Build history of the part. All positions in model axes, mm. Face numbers are marked on the shaded views. A direction names the side the tool comes from. Give positions to 0.01 mm unless a question says otherwise; leave off trailing zeros. Loops run counter-clockwise (first coordinate to the right, second up) from the corner with the lowest first, then second, coordinate; pieces in that order, holes last. Notation, with made-up numbers: (-33.5, 4.5) -> (14.5, 4.5) arc R26 ccw to (14.5, 24.5) -> close; hole circle Ø4 at (77, -1). An arc over 180 degrees is marked (long way). Answer in a Markdown table with one row per item. Add a question column.
from build123d import *

# Parameters (mm, degrees)
DODANIE_WYCI_GNI_CIE4_DEPTH = 13
SZKIC4_W                    = 21
SZKIC4_H                    = 13
DODANIE_WYCI_GNI_CIE5_DEPTH = 2
SZKIC5_W                    = 21
SZKIC5_H                    = 13
SZKIC5_R                    = 3
DODANIE_WYCI_GNI_CIE6_DEPTH = 4
DODANIE_WYCI_GNI_CIE7_START = -4
SZKIC5_4_R                  = 3
DODANIE_WYCI_GNI_CIE7_DEPTH = 3.6
ZAOKR_GLENIE3_R             = 8


with BuildPart() as part:
    # Szkic3 → Dodanie-wyci_gni_cie4 (new body)
    with BuildSketch(Plane(origin=(0, 0, 0), x_dir=(1, 0, 0), z_dir=(0, 1, 0))):
        Polygon((7.923824764, -2), (7.923824764, -0.6), (5.016097838, -0.6), (2.807764504, 1.65), (-3.360114975, 1.65), (-5.568448309, -0.6), (-8.476175236, -0.6), (-8.476175236, -2), (-10.5, -2), (-10.5, 2), (10.5, 2), (10.5, -2), align=None)
    extrude(amount=DODANIE_WYCI_GNI_CIE4_DEPTH)

    # Szkic4 → Dodanie-wyci_gni_cie5 (add)
    with BuildSketch(Plane(origin=(0, 0, -2), x_dir=(-1, 0, 0), z_dir=(0, 0, -1))):
        with Locations((0, 6.5)):
            Rectangle(SZKIC4_W, SZKIC4_H)
    extrude(amount=DODANIE_WYCI_GNI_CIE5_DEPTH)

    # Szkic5 → Dodanie-wyci_gni_cie6 (add)
    with BuildSketch(Plane(origin=(0, 0, -4), x_dir=(-1, 0, 0), z_dir=(0, 0, -1))):
        with Locations((0, 19.5)):
            Rectangle(SZKIC5_W, SZKIC5_H)
        with Locations((0, 20)):
            Circle(SZKIC5_R, mode=Mode.SUBTRACT)
        with Locations((0, -6.5)):
            Rectangle(SZKIC5_W, SZKIC5_H)
        with Locations((0, -7)):
            Circle(SZKIC5_R, mode=Mode.SUBTRACT)
    extrude(amount=-DODANIE_WYCI_GNI_CIE6_DEPTH)

    # Szkic5_4 → Dodanie-wyci_gni_cie7 (add)
    with BuildSketch(Plane(origin=(0, 0, -4), x_dir=(-1, 0, 0), z_dir=(0, 0, -1)).offset(DODANIE_WYCI_GNI_CIE7_START)):
        with BuildLine():
            Line((3, 16), (-3, 16))
            ThreePointArc((-3, 16), (0, 15), (3, 16))
        make_face()
        with BuildLine():
            ThreePointArc((5, 20), (-2.236067977, 24.472135955), (-3, 16))
            Line((-3, 16), (3, 16))
            ThreePointArc((3, 16), (4.472135955, 17.763932023), (5, 20))
        make_face()
        with Locations((0, 20)):
            Circle(SZKIC5_4_R, mode=Mode.SUBTRACT)
        with BuildLine():
            Line((-3, -3), (3, -3))
            ThreePointArc((3, -3), (0, -2), (-3, -3))
        make_face()
        with BuildLine():
            ThreePointArc((5, -7), (4.472135955, -4.763932023), (3, -3))
            Line((3, -3), (-3, -3))
            ThreePointArc((-3, -3), (-2.236067977, -11.472135955), (5, -7))
        make_face()
        with Locations((0, -7)):
            Circle(SZKIC5_4_R, mode=Mode.SUBTRACT)
    extrude(amount=-DODANIE_WYCI_GNI_CIE7_DEPTH)

    # Zaokr_glenie3
    zaokr_glenie3_edges = [part.edges().sort_by_distance(p)[0] for p in [
        (-10.5, -13, -2),
        (10.5, -13, -2),
        (10.5, 26, -2),
        (-10.5, 26, -2),
    ]]
    fillet(zaokr_glenie3_edges, radius=ZAOKR_GLENIE3_R)


solid = part.part
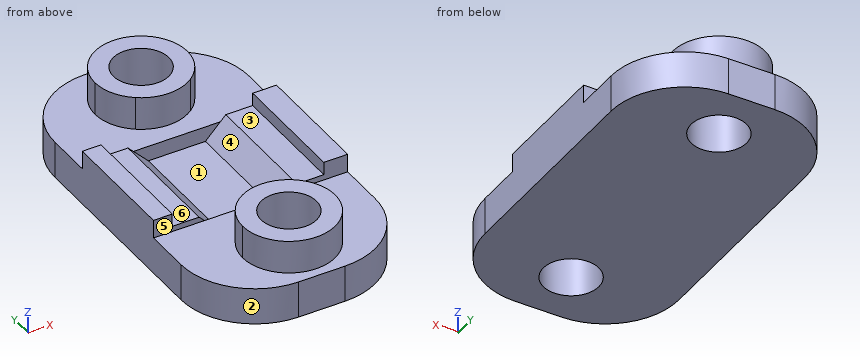
(1) Saw through at B-B, the plane x = 0. List the corners of the cut face in (y, z).
(2) 3-axis set-ups, long thin cutter, end or side, ignore diameter. For the marked faces 4, 5 and 6: which of +Z, -Z, +X, -X, +Y, -Y reach the whole face in a straight line?
(3) Wall check: line 1 along Y through (x, z) = (0, 0.75); line 2 along Y through (x, z) = (0, -1.5); line 3 along Y through (x, z) = (-1.25, -2.25). Give the ranges that are in metal, low to high. Write a range as from..to.
(4) Saw through at C-C, the plane z = -2.5. List the corners of the cut face in (x, y).
(5) Two-plate mould, pull along Y, no slides. Class the marked faces 1, 2 and 3: released by +Y, released by -Y, zero draft, split by the parting line, or undercut.
(6) Saw through at A-A, the plane z = 1.25. List the corners of the cut face in (x, y), then the cut area to 3 significant figures.
(7) Saw through at D-D, the plane y = -6. List the corners of the cut face in (x, z), then the cut area to 3 significant figures.
(8) Flat gauge pins, fed straight in: pin 1 Ø9.5 at (x, y) = (0, 20) entering from +Z; pin 2 Ø3 at (x, z) = (7, 2) entering from -Y; pin 3 Ø2 at (y, z) = (-9, -0.5) entering from -X; pin 4 Ø1.5 at (x, y) = (6, 5.5) entering from +Z. Where does each tip first touch, or does it go through?
Worked answers:
| question | item | result |
|---|---|---|
| 1 | outline | (-13, -4) -> (-10, -4) -> (-10, 3.6) -> (-12, 3.6) -> (-12, 0) -> (-13, 0) -> close; (-4, -4) -> (17, -4) -> (17, 3.6) -> (15, 3.6) -> (15, 0) -> (13, 0) -> (13, -1.65) -> (0, -1.65) -> (0, 0) -> (-2, 0) -> (-2, 3.6) -> (-4, 3.6) -> close; (23, -4) -> (26, -4) -> (26, 0) -> (25, 0) -> (25, 3.6) -> (23, 3.6) -> close |
| 2 | face 4 | +Z |
| 2 | face 5 | +Z, +X, -X, -Y |
| 2 | face 6 | +Z, +Y, -Y |
| 3 | line 1 | -12..-10, -4..-2, 15..17, 23..25 |
| 3 | line 2 | -13..-10, -4..0, 13..17, 23..26 |
| 3 | line 3 | -13..-9.73, -4.27..17.27, 22.73..26 |
| 4 | outline | (-10.5, -5) arc R8 ccw to (-2.5, -13) -> (2.5, -13) arc R8 ccw to (10.5, -5) -> (10.5, 18) arc R8 ccw to (2.5, 26) -> (-2.5, 26) arc R8 ccw to (-10.5, 18) -> close; hole circle Ø6 at (0, -7); hole circle Ø6 at (0, 20) |
| 5 | face 1 | undercut |
| 5 | face 2 | released by -Y |
| 5 | face 3 | zero draft |
| 6 | outline | (-10.5, 0) -> (-8.48, 0) -> (-8.48, 13) -> (-10.5, 13) -> close; circle Ø10 at (0, -7); circle Ø10 at (0, 20); (7.92, 0) -> (10.5, 0) -> (10.5, 13) -> (7.92, 13) -> close; hole circle Ø6 at (0, -7); hole circle Ø6 at (0, 20) |
| 6 | area | 160 mm^2 |
| 7 | outline | (-10.44, -4) -> (-2.83, -4) -> (-2.83, 3.6) -> (-4.9, 3.6) -> (-4.9, 0) -> (-10.44, 0) -> close; (2.83, -4) -> (10.44, -4) -> (10.44, 0) -> (4.9, 0) -> (4.9, 3.6) -> (2.83, 3.6) -> close |
| 7 | area | 75.8 mm^2 |
| 8 | pin 1 | z = 3.6 |
| 8 | pin 2 | y = 0 |
| 8 | pin 3 | x = -9.92 |
| 8 | pin 4 | z = 0.6 |
